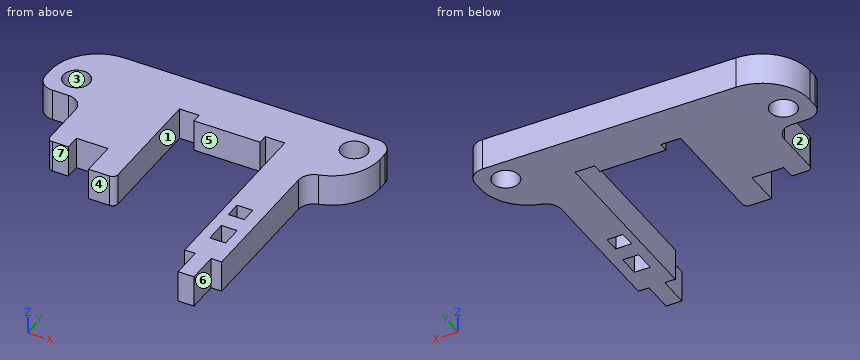
Autodesk Inventor part; units mm, degrees
ref_plane "YZ Plane" through (0, 0, 0) normal (1, 0, 0) x (0, 1, 0)
ref_plane "XZ Plane" through (0, 0, 0) normal (0, 1, 0) x (-1, 0, 0)
ref_plane "XY Plane" through (0, 0, 0) normal (0, 0, 1) x (1, 0, 0)
sketch "Sketch1" plane through (0, 0, 0) normal (0, 0, 1) x (1, 0, 0)
  line L0 (0, 4.25) -> (0, 7)
  line L1 (0, 7) -> (6, 7)
  line L2 (6, 7) -> (6, 0.3)
  line L3 (6, 0.3) -> (11, 0.3)
  line L4 (11, 0.3) -> (11, 22.5)
  line L5 (-4, 4.25) -> (0, 4.25)
  line L6 (30.939, 22.5) -> (27.2275, 22.5)
  line L7 (27.2275, 22.5) -> (27.2275, 20.708)
  line L8 (27.2275, 20.708) -> (14.7135, 20.708)
  line L9 (14.7135, 20.708) -> (14.7135, 22.5)
  line L10 (14.7135, 22.5) -> (11, 22.5)
  line L11 (30.939, 22.5) -> (30.939, -12)
  line L12 (30.939, -12) -> (32.939, -12)
  line L13 (32.939, -12) -> (32.939, -17.9)
  line L14 (32.939, -17.9) -> (35.939, -17.9)
  line L15 (35.939, -17.9) -> (35.939, -12)
  line L16 (35.939, -12) -> (37.939, -12)
  line L17 (37.939, -12) -> (37.939, 17)
  line L18 (37.939, 17) -> (46.9695, 17)
  line L19 (46.9695, 17) -> (46.9695, 30.708)
  line L20 (-4, 4.25) -> (-4, 17)
  line L21 (-4, 17) -> (-13.0305, 17)
  line L22 (-13.0305, 17) -> (-13.0305, 30.708)
  line L23 (46.9695, 30.708) -> (-13.0305, 30.708)
  dimension "d0" = 6
  dimension "d1" = 6.7
  dimension "d3" = 5
  dimension "d10" = 4
  dimension "d12" = 2.75
  dimension "d15" = 1.792
  dimension "d20" = 3
  dimension "d21" = 2
  dimension "d22" = 5.9
  dimension "d23" = 12.514
  dimension "d24" = 19.939
  dimension "d25" = 3.7135
  dimension "d42" = 13.708
  dimension "d43" = 19
  dimension "d48" = 7
  dimension "d50" = 60
  dimension "d51" = 41.939
  dimension "d52" = 9.0305
  dimension "d65" = 10
  dimension "d66" = 29
extrude "Extrusion1" add sketch "Sketch1" along normal blind 6
sketch "Sketch2" plane through (0, 0, 6) normal (0, 0, 1) x (1, 0, 0)
  line L0 (35.45, 0.264) -> (32.45, 0.264)
  line L1 (32.45, 0.264) -> (32.45, 3.264)
  line L2 (32.45, 3.264) -> (35.45, 3.264)
  line L3 (35.45, 3.264) -> (35.45, 0.264)
  line L4 (34.939, 35.708) -> (-1, 35.708)
  line L5 (30.939, 22.5) -> (30.939, -12)
  line L6 (32.939, -17.9) -> (35.939, -17.9)
  point P0 (0, 0)
  dimension "d26" = 3
  dimension "d27" = 3
  dimension "d61" = 18.164
  dimension "d62" = 1.511
extrude "Extrusion2" cut sketch "Sketch2" against normal blind 10
sketch "Sketch3" plane through (0, 0, 0) normal (0, 0, -1) x (-1, 0, 0)
  line L0 (-32.939, -7) -> (-35.939, -7)
  line L1 (-35.939, -7) -> (-35.939, -3)
  line L2 (-35.939, -3) -> (-32.939, -3)
  line L3 (-32.939, -3) -> (-32.939, -7)
  line L4 (-35.939, -12) -> (-37.939, -12)
  line L5 (-37.939, -12) -> (-37.939, 17)
  point P0 (0, 0)
  dimension "d32" = 3
  dimension "d33" = 4
  dimension "d34" = 5
  dimension "d63" = 2
extrude "Extrusion3" cut sketch "Sketch3" against normal blind 10
fillet "Fillet4" radius 1 2 edges at (11, 0.3, 3) (-4, 4.25, 3)
sketch "Sketch4" plane through (0, 0, 6) normal (0, 0, 1) x (1, 0, 0)
  circle A0 centre (41.9595, 26.3) radius 2.5
  circle A1 centre (-8.0305, 21.7) radius 2.5
  line L0 (-13.0305, 30.708) -> (-13.0305, 17)
  line L1 (-13.0305, 17) -> (-4, 17)
  line L2 (46.9695, 17) -> (46.9695, 30.708)
  line L3 (37.939, 17) -> (46.9695, 17)
  point P0 (0, 0)
  dimension "d45" = 5
  dimension "d46" = 5
  dimension "d53" = 5
  dimension "d67" = 4.7
  dimension "d70" = 5.01
  dimension "d71" = 9.3
extrude "Extrusion4" cut sketch "Sketch4" against normal blind 10
fillet "Fillet6" radius 9 2 edges at (-13.0305, 30.708, 3) (46.9695, 17, 3)
fillet "Fillet7" radius 3 4 edges at (37.939, 17, 3) (46.9695, 30.708, 3) (-4, 17, 3) (-13.0305, 17, 3)
properties part number "Gripper V 10.1 servo bracket bottom 6mm"
Design review of the part built by this model. Coordinates are the model's own, in mm. Face numbers are marked on the shaded views. A direction names the side the tool comes from. Round coordinates to 2 decimals unless told otherwise and drop trailing zeros. Loops run counter-clockwise (first coordinate to the right, second up) from the corner with the lowest first, then second, coordinate; pieces in that order, holes last. Notation, with made-up numbers: M -8.75,3.5 L 15.25,3.5 A37 cw 15.25,41.5 Z; hole C 84.5,20 d10. An arc over 180 degrees is marked long. Answer as a JSON object with one key per item and string values.
Item 1: Clearance check with flat-ended pins moving along their axes: P1, Ø2, axis at y = 12.5, z = 1.5, coming from the -X side; P2, Ø2, axis at y = 21.5, z = 3, coming from the +X side; P3, Ø3, axis at y = -2.5, z = 2.5, coming from the -X side; P4, Ø12, axis at x = 12, y = -7.5, coming from the -Z side. State where each tip first meets the part, or that it passes through.
Answer sheet:
{"P1": "stops at x = -4", "P2": "stops at x = 46.26", "P3": "stops at x = 30.94", "P4": "passes through"}
Item 2: We need section B-B on z = 2. State how many separate pieces and enclosed holes the cut face has, and give its area (3 significant figures).
Answer sheet:
{"separate pieces": "1", "enclosed holes": "4", "area": "1,050 mm^2"}
Item 3: Wall thickness on L1, parallel to X at y = 2.5, z = 4; L2, parallel to X at y = -6.5, z = 2.75; L3, parallel to X at y = 13, z = 5.75: over which ranges is each line inside the solid? List them lowest first. Write a range as from..to.
Answer sheet:
{"L1": "x = 6..11, 30.94..32.45, 35.45..37.94", "L2": "x = 30.94..32.94, 35.94..37.94", "L3": "x = -4..11, 30.94..37.94"}
Item 4: We need section C-C on x = 25. Give the boundary of the cut face in (y, z).
Answer sheet:
{"outline": "M 20.71,0 L 30.71,0 L 30.71,6 L 20.71,6 Z"}
Item 5: The part is to be moulded in two halves that separate along X. For the marked faces 1, 2, 3 and 4, say which applies: pulls with the +X half, pulls with the -X half, needs draft (parallel to the pull), parting line crosses it, or undercut.
Answer sheet:
{"face 1": "undercut", "face 2": "pulls with the -X half", "face 3": "undercut", "face 4": "needs draft"}
Item 6: Machinability: for the marked faces 5, 6 and 7, which of the approach directions +Z, -Z, +X, -X, +Y, -Y give a long, thin tool a straight path to every point of the face, cutting with its end or side? Answer none if there is none.
Answer sheet:
{"face 5": "+Z, -Z, -Y", "face 6": "+Z, -Z, +X, -Y", "face 7": "+Z, -Z, -X, -Y"}
Item 7: We need section A-A on y = -4.5. Give the boundary of the cut face in (x, z).
Answer sheet:
{"outline": "M 30.94,0 L 32.94,0 L 32.94,6 L 30.94,6 Z; M 35.94,0 L 37.94,0 L 37.94,6 L 35.94,6 Z"}
